Can you work these out from the model? Positions are in its coordinate system, mm. A direction names the side the tool comes from. Coordinates: 2 decimals unless noted, no trailing zeros. Order: outer loops, then holes, each group sorted by start corner. A loop starts at its lowest first (then second) coordinate and runs counter-clockwise, first axis right, second up. Notation, with made-up numbers: (36.5, -10.75) -> (44.5, -10.75) arc R24 cw to (44.5, 0.25) -> close; hole circle Ø6 at (24, 1.25). An arc over 180 degrees is marked (long way). Answer in a Markdown table with one row per item.
```python
from build123d import *

# Parameters (mm, degrees)
SKETCH1_W           = 567.538044716
SKETCH1_H           = 567.538044716
SKETCH1_W_2         = 80.467
SKETCH1_H_2         = 448.005044716
SKETCH1_W_3         = 45
SKETCH1_H_3         = 45
SKETCH1_W_4         = 448.005044716
SKETCH1_W_5         = 22.445
SKETCH1_H_4         = 22.445
SKETCH1_H_5         = 80.467
BOSS_EXTRUDE1_DEPTH = 13.022
SKETCH2_R           = 28.6
BOSS_EXTRUDE2_DEPTH = 110


with BuildPart() as part:
    # Sketch1 → Boss-Extrude1 (new body)
    with BuildSketch(Plane(origin=(0, 0, 0), x_dir=(1, 0, 0), z_dir=(0, 1, 0))):
        with Locations((283.769022358, 283.769022358)):
            Rectangle(SKETCH1_W, SKETCH1_H)
        with Locations((53.2555, 237.024522358)):
            Rectangle(SKETCH1_W_2, SKETCH1_H_2, mode=Mode.SUBTRACT)
        with Locations((35.522, 532.016044716)):
            Rectangle(SKETCH1_W_3, SKETCH1_H_3, mode=Mode.SUBTRACT)
        with Locations((330.513522358, 237.024522358)):
            Rectangle(SKETCH1_W_4, SKETCH1_H_2, mode=Mode.SUBTRACT)
        with Locations((82.2665, 532.016044716)):
            Rectangle(SKETCH1_W_5, SKETCH1_H_3, mode=Mode.SUBTRACT)
        with Locations((35.522, 485.271544716)):
            Rectangle(SKETCH1_W_3, SKETCH1_H_4, mode=Mode.SUBTRACT)
        with Locations((330.513522358, 514.282544716)):
            Rectangle(SKETCH1_W_4, SKETCH1_H_5, mode=Mode.SUBTRACT)
        with Locations((82.2665, 485.271544716)):
            Rectangle(SKETCH1_W_5, SKETCH1_H_4, mode=Mode.SUBTRACT)
    extrude(amount=BOSS_EXTRUDE1_DEPTH)

    # Sketch2 → Boss-Extrude2 (add)
    with BuildSketch(Plane.XZ):
        with Locations(Location((64.533, -503.005044716, 0), (0, 0, 103.159188844))):
            Circle(SKETCH2_R)
    extrude(amount=BOSS_EXTRUDE2_DEPTH)


solid = part.part
```
(1) Suppose I cut it at A-A (z = -47.5). Please give me the cut outline in (x, y).
Response values:
| item | result |
|---|---|
| outline | (0, 0) -> (13.02, 0) -> (13.02, 13.02) -> (0, 13.02) -> close; (93.49, 0) -> (106.51, 0) -> (106.51, 13.02) -> (93.49, 13.02) -> close; (554.52, 0) -> (567.54, 0) -> (567.54, 13.02) -> (554.52, 13.02) -> close |
(2) Will these pins go through, and if not, where does the flat tip stop? pin 1 Ø14.5 at (x, y) = (68, 8.5) entering from +Z; pin 2 Ø3 at (y, z) = (-96.5, -472.5) entering from -X (3 decimals); pin 3 Ø6.5 at (x, z) = (77.5, -486) entering from +Y.
Response values:
| item | result |
|---|---|
| pin 1 | z = 0 |
| pin 2 | through |
| pin 3 | y = 0 |
(3) Suppose I cut it at C-C (y = -81.5). Please give me the cut outline in (x, z), and give its area (3 significant figures).
Response values:
| item | result |
|---|---|
| outline | circle Ø57.2 at (64.53, -503.01) |
| area | 2,570 mm2 |
(4) I need wall thicknesses on line 1 (Z direction, x = 315, y = 4.5). Which ranges of the line are inside material? Lowest first, please. Write a range as [from, to].
Response values:
| item | result |
|---|---|
| line 1 | [-567.54, -554.52], [-474.05, -461.03], [-13.02, 0] |
(5) On a 3-axis mill with a long thin cutter (end or side, diameter ignored), from which of +Z, -Z, +X, -X, +Y, -Y can I reach the whole of each face in a straight line? I mean faces 1 (the flat face through (554.516, 6, -234)), 2 (the flat face through (78, 0, -519)), 3 (the flat face through (64, -110, -503)). Say none if no direction works.
Response values:
| item | result |
|---|---|
| face 1 | +Y, -Y |
| face 2 | +Y |
| face 3 | +Z, -Z, +X, -X, -Y |
(6) We'd pull the mould along Z, two halves only. Please class faces 4 (the flat face through (327, 6, -474.049)), 5 (the flat face through (567.538, 6, -280)), 6 (the cylindrical face through (37.77, -54.23, -513.09)): +Z half, -Z half, draft (parallel to the pull), parting line (faces both ways), or undercut.
Response values:
| item | result |
|---|---|
| face 4 | undercut |
| face 5 | draft |
| face 6 | parting line |
(7) Suppose I cut it at B-B (x = 528.5). Please give me the cut outline in (y, z), and give its area (3 significant figures).
Response values:
| item | result |
|---|---|
| outline | (0, -567.54) -> (13.02, -567.54) -> (13.02, -554.52) -> (0, -554.52) -> close; (0, -474.05) -> (13.02, -474.05) -> (13.02, -461.03) -> (0, -461.03) -> close; (0, -13.02) -> (13.02, -13.02) -> (13.02, 0) -> (0, 0) -> close |
| area | 509 mm2 |
